Read the model definition and answer for the solid it produces. Units are mm, in the model's axes. A direction names the side the tool comes from. Give positions to 0.01 mm unless a question says otherwise; leave off trailing zeros. Order: outer loops, then holes, each group sorted by start corner. A loop starts at its lowest first (then second) coordinate and runs counter-clockwise, first axis right, second up. Notation, with made-up numbers: M 55,25 L 61,25 A17 ccw 61,38 Z; hole C 75,73 d3. An arc over 180 degrees is marked long. One line per item, written item: value.
from build123d import *

# Parameters (mm, degrees)
SKETCH1_W           = 125.7
SKETCH1_H           = 125.7
BOSS_EXTRUDE1_DEPTH = 376.8
SKETCH3_W           = 83
SKETCH3_H           = 364.1
CUT_EXTRUDE1_DEPTH  = 126.35
SKETCH5_W           = 83
SKETCH5_H           = 364.1
CUT_EXTRUDE2_DEPTH  = 126.35


with BuildPart() as part:
    # Sketch1 → Boss-Extrude1 (new body)
    with BuildSketch(Plane(origin=(0, 0, 0), x_dir=(1, 0, 0), z_dir=(0, 1, 0))):
        Rectangle(SKETCH1_W, SKETCH1_H)
        Polygon((-47.5, -56.5), (-47.5, -50), (-41.5, -50), (-41.5, -56.5), (41.5, -56.5), (41.5, -50), (47.5, -50), (47.5, -56.5), (56.5, -56.5), (56.5, -47.5), (50, -47.5), (50, -41.5), (56.5, -41.5), (56.5, 41.5), (50, 41.5), (50, 47.5), (56.5, 47.5), (56.5, 56.5), (47.5, 56.5), (47.5, 50), (41.5, 50), (41.5, 56.5), (-41.5, 56.5), (-41.5, 50), (-47.5, 50), (-47.5, 56.5), (-56.5, 56.5), (-56.5, 47.5), (-50, 47.5), (-50, 41.5), (-56.5, 41.5), (-56.5, -41.5), (-50, -41.5), (-50, -47.5), (-56.5, -47.5), (-56.5, -56.5), align=None, mode=Mode.SUBTRACT)
    extrude(amount=BOSS_EXTRUDE1_DEPTH)

    # Sketch3 → Cut-Extrude1 (cut)
    with BuildSketch(Plane(origin=(62.85, 0, 0), x_dir=(0, 0, -1), z_dir=(1, 0, 0))):
        with Locations((0, 188.4)):
            Rectangle(SKETCH3_W, SKETCH3_H)
    extrude(amount=-CUT_EXTRUDE1_DEPTH, mode=Mode.SUBTRACT)

    # Sketch5 → Cut-Extrude2 (cut)
    with BuildSketch(Plane.XY.offset(62.85)):
        with Locations((0, 188.4)):
            Rectangle(SKETCH5_W, SKETCH5_H)
    extrude(amount=-CUT_EXTRUDE2_DEPTH, mode=Mode.SUBTRACT)


solid = part.part
1) Which of the six approach directions +Z, -Z, +X, -X, +Y, -Y give full straight-line access (tool end or side, diameter ignored) to faces 1 (the face through (60, 370.45, 1)), 2 (the face through (-5, 0, 60)), 3 (the face through (53, 186, -47.5))?
Reported:
face 1: +X, -X
face 2: +Z, -Z, +X, -X, -Y
face 3: +Y, -Y
2) Find section B-B, the plane z = 36. Write down the section's boundary in (x, y).
Reported:
outline: M -62.85,0 L -56.5,0 L -56.5,6.35 L -62.85,6.35 Z; M -62.85,370.45 L -56.5,370.45 L -56.5,376.8 L -62.85,376.8 Z; M 56.5,0 L 62.85,0 L 62.85,6.35 L 56.5,6.35 Z; M 56.5,370.45 L 62.85,370.45 L 62.85,376.8 L 56.5,376.8 Z
3) Consider probe 1 along X at (y, z) = (73, 52); probe 2 along Z at (x, y) = (-49, 45). Determine where each line is inside the solid, lowest interval first.
Reported:
probe 1: x = -62.85 to -56.5, -47.5 to -41.5, 41.5 to 47.5, 56.5 to 62.85
probe 2: z = -62.85 to -56.5, 56.5 to 62.85
4) This flat-tipped pin is pushed along its axis until it touches: pin 1 Ø6 at (x, y) = (-37.5, 200.5) entering from +Z. Where does it stop, or does it pass through?
Reported:
pin 1: passes through
5) Find section C-C, the plane y = 273.5. Count the separate pieces of the cut face and the enclosed holes in it, plus the area to 3 significant figures.
Reported:
separate pieces: 4
enclosed holes: 0
area: 1,240 mm^2
6) Find section A-A, the plane x = 22. Write down the section's boundary in (y, z), plus the area to 3 significant figures.
Reported:
outline: M 0,-62.85 L 6.35,-62.85 L 6.35,-56.5 L 0,-56.5 Z; M 0,56.5 L 6.35,56.5 L 6.35,62.85 L 0,62.85 Z; M 370.45,-62.85 L 376.8,-62.85 L 376.8,-56.5 L 370.45,-56.5 Z; M 370.45,56.5 L 376.8,56.5 L 376.8,62.85 L 370.45,62.85 Z
area: 161 mm^2
7) Determine the mould class of faces 4 (the face through (62.85, 174, 42)), 5 (the face through (-1, 370.45, 60)), 6 (the face through (-42, 174, 62.85)), 7 (the face through (-1, 6.35, -60)) for opening direction X: +X half, -X half, draft (parallel to the pull), parting line (faces both ways), or undercut.
Reported:
face 4: +X half
face 5: undercut
face 6: draft
face 7: undercut
